Work out the finished part from the listing and answer in its coordinate system (mm). Face numbers are marked on the shaded views. A direction names the side the tool comes from. Give positions to 0.01 mm unless a question says otherwise; leave off trailing zeros. Write each loop counter-clockwise with the first axis right and the second up, starting at its lowest first coordinate (ties: lowest second). Pieces come first, ordered by that corner, then holes. Notation, with made-up numbers: (49.25, 52) -> (87.25, 52) arc R20 cw to (87.25, 58) -> close; hole circle Ø4 at (-2, 2). An arc over 180 degrees is marked (long way). Use a Markdown table: item, result. Add a question column.
Q1. For a pull along Y with two mould halves and no side action, classify the marked faces 3 and 4 as pulls with the +Y half, pulls with the -Y half, needs draft (parallel to the pull), parting line crosses it, or undercut.
Q2. Consider line 1 (Y direction, x = 3, z = 0); line 2 (Y direction, x = -37, z = 0); line 3 (Z direction, x = -48, y = -47.5). Determine where each line is inside the solid, lowest interval first.
Q3. Section B-B, the plane z = 0 is taken. Give the vertices of the cut face in (x, y), plus the area to 3 significant figures.
Q4. For the marked faces 1 and 2, determine the directions among +Z, -Z, +X, -X, +Y, -Y from which every point of the face is accessible in a straight line to the end or side of a thin tool.
Q5. Section C-C, the plane x = 9.5 is taken. Give the vertices of the cut face in (y, z), plus the area to 3 significant figures.
Q6. Section A-A, the plane y = 0 is taken. Give the vertices of the cut face in (x, z).
Q7. Section D-D, the plane y = -20 is taken. Give the vertices of the cut face in (x, z), plus the area to 3 significant figures.
Q8. Each of these flat-tipped pins is pushed along its axis until it touches: pin 1 Ø5 at (y, z) = (-43, 25) entering from -X; pin 2 Ø10 at (y, z) = (-41.5, 22.5) entering from +X; pin 3 Ø1.5 at (x, z) = (-132, -52) entering from +Y; pin 4 Ø4 at (x, y) = (16, 0) entering from -Z. Where does it stop, or does it pass through?
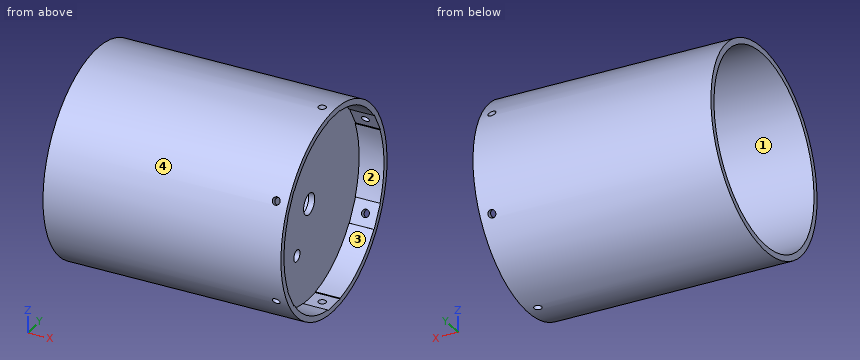
from build123d import *

# Parameters (mm, degrees)
SZKIC1_W                   = 5
SZKIC1_H                   = 5
SZKIC1_W_2                 = 21
SZKIC1_W_3                 = 175.265013497
SZKIC1_H_2                 = 81.5
SZKIC7_R                   = 3.25
WYTNIJ_WYCI_GNI_CIE1_DEPTH = 100
SZYK_KO_OWY1_COUNT         = 6
WYTNIJ_WYCI_GNI_CIE3_DEPTH = 21
SZYK_KO_OWY2_COUNT         = 6
WYTNIJ_WYCI_GNI_CIE2_REACH = 219.853
SZKIC8_R                   = 9
SZKIC8_R_2                 = 5


with BuildPart() as part:
    # Szkic1 → Obrót1 (revolve)
    with BuildSketch(Plane.XY, mode=Mode.PRIVATE) as obr_t1_sk:
        with Locations((2.5, 84)):
            Rectangle(SZKIC1_W, SZKIC1_H)
        with Locations((15.5, 84)):
            Rectangle(SZKIC1_W_2, SZKIC1_H)
        with Locations((-87.632506749, 84)):
            Rectangle(SZKIC1_W_3, SZKIC1_H)
        with Locations((2.5, 40.75)):
            Rectangle(SZKIC1_W, SZKIC1_H_2)
    revolve(obr_t1_sk.sketch.rotate(Axis((5, 0, 0), (-1, 0, 0)), 90), axis=Axis((5, 0, 0), (-1, 0, 0)))

    # Szkic7 → Wytnij-wyciągnięcie1 (cut)
    with BuildSketch(Plane.XY):
        with Locations(Location((16, 0, 0), (0, 0, 180))):
            Circle(SZKIC7_R)
    wytnij_wyci_gni_cie1 = extrude(amount=WYTNIJ_WYCI_GNI_CIE1_DEPTH, mode=Mode.SUBTRACT)

    # Szyk kołowy1: Wytnij-wyciągnięcie1 ×6 about axis
    szyk_ko_owy1_axis = Axis((26, 0, 0), (1, 0, 0))
    for i in range(1, SZYK_KO_OWY1_COUNT):
        add(wytnij_wyci_gni_cie1.rotate(szyk_ko_owy1_axis, i * 360 / SZYK_KO_OWY1_COUNT), mode=Mode.SUBTRACT)

    # Szkic9 → Wytnij-wyciągnięcie3 (cut)
    with BuildSketch(Plane(origin=(26, 0, 0), x_dir=(0, 0, -1), z_dir=(1, 0, 0))):
        Polygon((-81.5, 0), (-81.5, 10.1), (-77.682544911, 10.1), (-77.682544911, -10.1), (-81.5, -10.1), align=None)
    wytnij_wyci_gni_cie3 = extrude(amount=-WYTNIJ_WYCI_GNI_CIE3_DEPTH, mode=Mode.SUBTRACT)

    # Szyk kołowy2: Wytnij-wyciągnięcie3 ×6 about axis
    szyk_ko_owy2_axis = Axis((0, 0, 0), (1, 0, 0))
    for i in range(1, SZYK_KO_OWY2_COUNT):
        add(wytnij_wyci_gni_cie3.rotate(szyk_ko_owy2_axis, i * 360 / SZYK_KO_OWY2_COUNT), mode=Mode.SUBTRACT)

    # Szkic8 → Wytnij-wyciągnięcie2 (cut, up to next)
    with BuildSketch(Plane(origin=(5, 0, 0), x_dir=(0, 0, -1), z_dir=(1, 0, 0)), mode=Mode.PRIVATE) as wytnij_wyci_gni_cie2_sk1:
        Circle(SZKIC8_R)
    wytnij_wyci_gni_cie2_tool1 = extrude(wytnij_wyci_gni_cie2_sk1.sketch, amount=-WYTNIJ_WYCI_GNI_CIE2_REACH, mode=Mode.PRIVATE) & part.part
    # Szkic8 → Wytnij-wyciągnięcie2 (cut, up to next)
    with BuildSketch(Plane(origin=(5, 0, 0), x_dir=(0, 0, -1), z_dir=(1, 0, 0)), mode=Mode.PRIVATE) as wytnij_wyci_gni_cie2_sk2:
        with Locations((34.641016151, -20)):
            Circle(SZKIC8_R_2)
    wytnij_wyci_gni_cie2_tool2 = extrude(wytnij_wyci_gni_cie2_sk2.sketch, amount=-WYTNIJ_WYCI_GNI_CIE2_REACH, mode=Mode.PRIVATE) & part.part
    add(wytnij_wyci_gni_cie2_tool1.solids().sort_by_distance((5, 0, 0))[0], mode=Mode.SUBTRACT)
    add(wytnij_wyci_gni_cie2_tool2.solids().sort_by_distance((5, -20, -34.641016))[0], mode=Mode.SUBTRACT)


solid = part.part
Result set:
| question | item | result |
|---|---|---|
| 1 | face 3 | undercut |
| 1 | face 4 | parting line crosses it |
| 2 | line 1 | y = -86.5 to -9, 9 to 86.5 |
| 2 | line 2 | y = -86.5 to -81.5, 81.5 to 86.5 |
| 2 | line 3 | z = -72.29 to -66.23, 66.23 to 72.29 |
| 3 | outline | (-175.27, -86.5) -> (26, -86.5) -> (26, -81.5) -> (5, -81.5) -> (5, -9) -> (0, -9) -> (0, -81.5) -> (-175.27, -81.5) -> close; (-175.27, 81.5) -> (0, 81.5) -> (0, 9) -> (5, 9) -> (5, 81.5) -> (26, 81.5) -> (26, 86.5) -> (-175.27, 86.5) -> close |
| 3 | area | 2,740 mm2 |
| 4 | face 1 | -X |
| 4 | face 2 | +X |
| 5 | outline | circle Ø173 at (0, 0); hole (-75.63, -32) -> (-65.53, -49.5) -> (-64.99, -49.18) arc R81.5 ccw to (-10.1, -80.87) -> (-10.1, -81.5) -> (10.1, -81.5) -> (10.1, -80.87) arc R81.5 ccw to (64.99, -49.18) -> (65.53, -49.5) -> (75.63, -32) -> (75.09, -31.69) arc R81.5 ccw to (75.09, 31.69) -> (75.63, 32) -> (65.53, 49.5) -> (64.99, 49.18) arc R81.5 ccw to (10.1, 80.87) -> (10.1, 81.5) -> (-10.1, 81.5) -> (-10.1, 80.87) arc R81.5 ccw to (-64.99, 49.18) -> (-65.53, 49.5) -> (-75.63, 32) -> (-75.09, 31.69) arc R81.5 ccw to (-75.09, -31.69) -> close |
| 5 | area | 2,610 mm2 |
| 6 | outline | (-175.27, -86.5) -> (12.75, -86.5) -> (12.75, -81.5) -> (5, -81.5) -> (5, -9) -> (0, -9) -> (0, -81.5) -> (-175.27, -81.5) -> close; (-175.27, 81.5) -> (0, 81.5) -> (0, 9) -> (5, 9) -> (5, 81.5) -> (12.75, 81.5) -> (12.75, 86.5) -> (-175.27, 86.5) -> close; (19.25, -86.5) -> (26, -86.5) -> (26, -81.5) -> (19.25, -81.5) -> close; (19.25, 81.5) -> (26, 81.5) -> (26, 86.5) -> (19.25, 86.5) -> close |
| 7 | outline | (-175.27, -84.16) -> (26, -84.16) -> (26, -79.01) -> (5, -79.01) -> (5, -39.64) -> (0, -39.64) -> (0, -79.01) -> (-175.27, -79.01) -> close; (-175.27, 79.01) -> (0, 79.01) -> (0, -29.64) -> (5, -29.64) -> (5, 79.01) -> (26, 79.01) -> (26, 84.16) -> (-175.27, 84.16) -> close |
| 7 | area | 2,810 mm2 |
| 8 | pin 1 | stops at x = 0 |
| 8 | pin 2 | stops at x = 5 |
| 8 | pin 3 | stops at y = 69.68 |
| 8 | pin 4 | passes through |
